Geometry check sheet. Reference: the model listing, model coordinates, mm. Face numbers are marked on the shaded views. A direction names the side the tool comes from. Coordinates: 2 decimals unless noted, no trailing zeros. Loops run counter-clockwise (first coordinate to the right, second up) from the corner with the lowest first, then second, coordinate; pieces in that order, holes last. Notation, with made-up numbers: (-23.5, -25.75) - (-1.5, -25.75) arc R18 cw to (-1.5, -0.75) - close; hole circle Ø10 at (67, 56). An arc over 180 degrees is marked (long way). Write item = value, one per line. Start each with the question number.
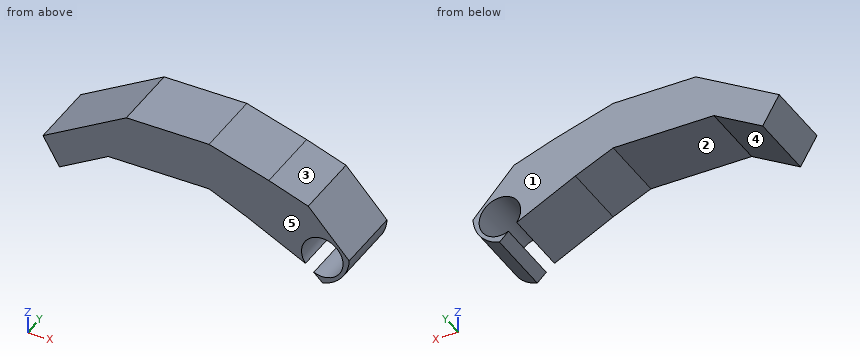
from build123d import *

# Parameters (mm, degrees)
F1_DEPTH = 12.7
F3_D     = 7.5946
F5_DEPTH = 25.4


with BuildPart() as f1:
    # F0 (on Front) → F1 (new body)
    with BuildSketch(Plane.XZ):
        Polygon((-18.419567, 0), (0, 0), (6.907339, -3.165863), (18.131765, -8.921978), (26.765935, -17.268345), (29.356185, -9.49759), (18.131765, 2.878058), (10.936619, 5.468309), (0, 8.845153), (-15.116255, 8.845153), (-30.349583, 0), (-27.34155, -5.180503), align=None)
    extrude(amount=F1_DEPTH)

    # F3 (through all)
    with Locations(Plane.XZ.offset(12.7)):
        with Locations((20.701887, -6.43437)):
            Hole(F3_D / 2)

    # F4 (on face) → F5 (cut)
    with BuildSketch(Plane.XZ.offset(12.7)):
        with BuildLine():
            ThreePointArc((25.619942, -5.378141), (24.214986, -9.235351), (20.777755, -11.47977))
            Line((20.777755, -11.47977), (26.765935, -17.268345))
            Line((26.765935, -17.268345), (29.356185, -9.49759))
            Line((29.356185, -9.49759), (25.619942, -5.378141))
        make_face()
    extrude(amount=-F5_DEPTH, mode=Mode.SUBTRACT)


solid = f1.part
(1) Sectioned sample at B-B on x = -9.5. Enter the section's corners in (y, z).
(2) Depth check by flat-ended pin: pin 1 (3 mm diameter, centred on y = -10.5, z = 4.5, fed in from -X); pin 2 (1.5 mm diameter, centred on x = -20, y = -11, fed in from -Z); pin 3 (2 mm diameter, centred on y = -2.5, z = -8.5, fed in from -X). Enter the tip coordinate at first touch or a pass-through.
(3) Sectioned sample at A-A on y = -9.75. Enter the section's corners in (x, z).
(4) Scan lines: line 1 (Z direction, x = -2.5, y = -2.5); line 2 (X direction, y = -8.5, z = -4.5); line 3 (X direction, y = -8.5, z = -2.25). Record each from-to range of solid material in increasing order.
(5) Tool access check on the marked faces 1 and 2. Record the directions out of +Z, -Z, +X, -X, +Y, -Y that give a thin tool (end or side, any length) a straight path to the whole face; none if there is none.
(6) Draft check along X on the marked faces 3, 4 and 5. Enter one of: pulls with the +X half, pulls with the -X half, needs draft (parallel to the pull), parting line crosses it, or undercut.
(7) Sectioned sample at C-C on z = 1.5. Enter the section's corners in (x, y).
Working result:
q1.outline = (-12.7, 0) - (0, 0) - (0, 8.85) - (-12.7, 8.85) - close
q2.pin_1 = -25.18
q2.pin_2 = -1.35
q2.pin_3 = 15.36
q3.outline = (-30.35, 0) - (-27.34, -5.18) - (-18.42, 0) - (0, 0) - (6.91, -3.17) - (17.63, -8.66) arc R3.8 cw (long way) to (19.14, -9.89) - (20.78, -11.48) arc R6.5 ccw to (25.62, -5.38) - (18.13, 2.88) - (10.94, 5.47) - (0, 8.85) - (-15.12, 8.85) - close
q4.line_1 = 0 to 8.85
q4.line_2 = -27.74 to -26.17, 9.51 to 17.43, 23.97 to 24.82
q4.line_3 = -29.04 to -22.29, 4.91 to 22.78
q5.face_1 = +Z, -Z, +X, -X, +Y
q5.face_2 = -Z, +Y, -Y
q6.face_3 = pulls with the +X half
q6.face_4 = undercut
q6.face_5 = needs draft
q7.outline = (-27.77, -12.7) - (19.38, -12.7) - (19.38, 0) - (-27.77, 0) - close
